Work out the finished part from the listing and answer in its coordinate system (mm). Face numbers are marked on the shaded views. Coordinates: 2 decimals unless noted, no trailing zeros. Loops run counter-clockwise (first coordinate to the right, second up) from the corner with the lowest first, then second, coordinate; pieces in that order, holes last. Notation, with made-up numbers: (-12.5, 43.5) -> (-7.5, 43.5) arc R17 cw to (-7.5, 54.5) -> close; hole circle Ø5 at (86, 80.25). An arc over 180 degrees is marked (long way). Use a Markdown table: item, result. Add a question column.
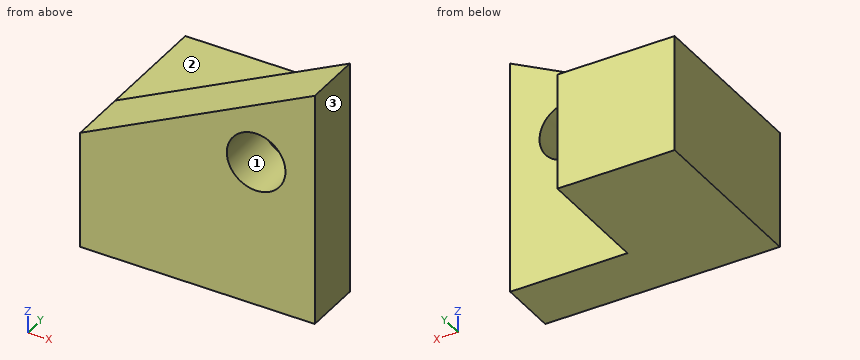
```python
from build123d import *

# Parameters (mm, degrees)
SKETCH1_W           = 1016
SKETCH1_H           = 1016
BOSS_EXTRUDE1_DEPTH = 1016
CUT_EXTRUDE1_DEPTH  = 1016
CUT_EXTRUDE2_DEPTH  = 762
SKETCH4_W           = 508
SKETCH4_H           = 254
CUT_EXTRUDE3_DEPTH  = 762
SKETCH5_R           = 127
CUT_EXTRUDE4_DEPTH  = 762


with BuildPart() as part:
    # Sketch1 → Boss-Extrude1 (new body)
    with BuildSketch(Plane(origin=(0, 0, 0), x_dir=(1, 0, 0), z_dir=(0, 1, 0))):
        with Locations((508, 508)):
            Rectangle(SKETCH1_W, SKETCH1_H)
    extrude(amount=BOSS_EXTRUDE1_DEPTH)

    # Sketch2 → Cut-Extrude1 (cut)
    with BuildSketch(Plane(origin=(0, 1016, 0), x_dir=(1, 0, 0), z_dir=(0, 1, 0))):
        Polygon((0, 0), (1016, 0), (0, 508), align=None)
    extrude(amount=-CUT_EXTRUDE1_DEPTH, mode=Mode.SUBTRACT)

    # Sketch3 → Cut-Extrude2 (cut)
    with BuildSketch(Plane(origin=(0, 1016, 0), x_dir=(1, 0, 0), z_dir=(0, 1, 0))):
        Polygon((0, 508), (508, 508), (508, 1016), (1016, 1016), (1016, 0), align=None)
    extrude(amount=-CUT_EXTRUDE2_DEPTH, mode=Mode.SUBTRACT)

    # Sketch4 → Cut-Extrude3 (cut)
    with BuildSketch(Plane.XY.offset(-508)):
        with Locations((254, 889)):
            Rectangle(SKETCH4_W, SKETCH4_H)
    extrude(amount=-CUT_EXTRUDE3_DEPTH, mode=Mode.SUBTRACT)

    # Sketch5 → Cut-Extrude4 (cut)
    with BuildSketch(Plane(origin=(0, 254, 0), x_dir=(1, 0, 0), z_dir=(0, 1, 0))):
        with Locations(Location((762, 381, 0), (0, 0, 270))):
            Circle(SKETCH5_R)
    extrude(amount=-CUT_EXTRUDE4_DEPTH, mode=Mode.SUBTRACT)


solid = part.part
```
Item 1: Section A-A (x = 762) is taken. Determine the outline of the cut face in (y, z), then the cut area to 3 significant figures.
Item 2: For a pull along Z with two mould halves and no side action, classify the marked faces 1, 2 and 3 as +Z half, -Z half, draft (parallel to the pull), parting line (faces both ways), or undercut.
Item 3: Find the intervals of material crossed by probe 1 along X at (y, z) = (200, -381); probe 2 along Y at (x, z) = (725, -735.5); probe 3 along X at (y, z) = (370, -793.5), in increasing order.
Item 4: Section D-D (x = 193.5) is taken. Determine the outline of the cut face in (y, z).
Item 5: Section C-C (y = 81) is taken. Determine the outline of the cut face in (x, z).
Item 6: Section B-B (z = -381) is taken. Determine the outline of the cut face in (x, y).
Item 7: Given pin 1 (1 mm diameter, centred on y = 229.5, z = -384, fed in from -X); pin 2 (10 mm diameter, centred on y = 135.5, z = -366.5, fed in from -X); pin 3 (5 mm diameter, centred on x = 173, z = -443.5, fed in from +Y); pin 4 (12 mm diameter, centred on x = 313, z = -508, fed in from -Y), each flat-ended and moving along its own axis, determine where each tip first touches the part or whether it passes through.
Output:
| question | item | result |
|---|---|---|
| 1 | outline | (0, -1016) -> (254, -1016) -> (254, -508) -> (0, -508) -> close; (0, -254) -> (254, -254) -> (254, -127) -> (0, -127) -> close |
| 1 | area | 161,000 mm2 |
| 2 | face 1 | undercut |
| 2 | face 2 | +Z half |
| 2 | face 3 | draft |
| 3 | probe 1 | x = 254 to 635, 889 to 1016 |
| 3 | probe 2 | y = 0 to 254 |
| 3 | probe 3 | x = 0 to 508 |
| 4 | outline | (0, -1016) -> (762, -1016) -> (762, -508) -> (254, -508) -> (254, -411.25) -> (0, -411.25) -> close |
| 5 | outline | (0, -1016) -> (1016, -1016) -> (1016, 0) -> (0, -508) -> close; hole circle Ø254 at (762, -381) |
| 6 | outline | (254, 0) -> (635, 0) -> (635, 254) -> (254, 254) -> close; (889, 0) -> (1016, 0) -> (1016, 254) -> (889, 254) -> close |
| 7 | pin 1 | stops at x = 247 |
| 7 | pin 2 | stops at x = 273 |
| 7 | pin 3 | stops at y = 254 |
| 7 | pin 4 | stops at y = 0 |
